Can you work these out from the model? Positions are in its coordinate system, mm. A direction names the side the tool comes from. Round coordinates to 2 decimals unless told otherwise and drop trailing zeros. Loops run counter-clockwise (first coordinate to the right, second up) from the corner with the lowest first, then second, coordinate; pieces in that order, holes last. Notation, with made-up numbers: (58, 23) -> (84, 23) arc R21 cw to (84, 60) -> close; hole circle Ø10 at (-2, 6). An arc over 180 degrees is marked (long way). Use a Markdown table: item, result.
from build123d import *

# Parameters (mm, degrees)
SKETCH_1_W          = 8
SKETCH_1_H          = 8
EXTRUDE_1_DEPTH     = 8
CUT_EXTRUDE_1_DEPTH = 8
SKETCH_3_R          = 3
EXTRUDE_2_DEPTH     = 60


with BuildPart() as part:
    # 草图1 → 凸台-拉伸1 (new body)
    with BuildSketch(Plane(origin=(0, 0, 0), x_dir=(1, 0, 0), z_dir=(0, 1, 0))):
        Rectangle(SKETCH_1_W, SKETCH_1_H)
    extrude(amount=EXTRUDE_1_DEPTH)

    # 草图2 → 切除-拉伸1 (cut)
    with BuildSketch(Plane.XY.offset(4)):
        with BuildLine():
            Line((-4, 4), (-4, 9.423328326))
            Line((-4, 9.423328326), (4, 9.423328326))
            Line((4, 9.423328326), (4, 4))
            ThreePointArc((4, 4), (0, 8), (-4, 4))
        make_face()
    extrude(amount=-CUT_EXTRUDE_1_DEPTH, mode=Mode.SUBTRACT)

    # 草图3 → 凸台-拉伸2 (add)
    with BuildSketch(Plane.XZ):
        Circle(SKETCH_3_R)
    extrude(amount=EXTRUDE_2_DEPTH)


solid = part.part
1. I need wall thicknesses on line 1 (Y direction, x = 0, z = 3.75); line 2 (Y direction, x = -0.25, z = -2.5); line 3 (Z direction, x = 1, y = -22.5). Which ranges of each line are inside material? Lowest first, please.
Answer sheet:
| item | result |
|---|---|
| line 1 | y = 0 to 8 |
| line 2 | y = -60 to 7.99 |
| line 3 | z = -2.83 to 2.83 |
2. Which directions (+Z, -Z, +X, -X, +Y, -Y) give clear straight access to the entire face, cutting with the end or side of a thin tool? Please do faces 1 (the flat face through (0, 4, -4)), 2 (the flat face through (2, 0, -3)).
Answer sheet:
| item | result |
|---|---|
| face 1 | -Z, +X, -X, +Y, -Y |
| face 2 | -Y |
3. I want a section at B-B (y = -48). Please give me the cut outline in (x, z).
Answer sheet:
| item | result |
|---|---|
| outline | circle Ø6 at (0, 0) |
4. I want a section at C-C (x = 0.75). Please give me the cut outline in (y, z).
Answer sheet:
| item | result |
|---|---|
| outline | (-60, -2.9) -> (0, -2.9) -> (0, -4) -> (7.93, -4) -> (7.93, 4) -> (0, 4) -> (0, 2.9) -> (-60, 2.9) -> close |
5. Will these pins go through, and if not, where does the flat tip stop? pin 1 Ø3 at (x, y) = (2, -35.5) entering from -Z; pin 2 Ø1 at (x, y) = (3, -49.5) entering from -Z.
Answer sheet:
| item | result |
|---|---|
| pin 1 | stops at z = -2.96 |
| pin 2 | stops at z = -1.66 |
6. I want a section at A-A (z = 0). Please give me the cut outline in (x, y), plus the area to 3 significant figures.
Answer sheet:
| item | result |
|---|---|
| outline | (-4, 0) -> (-3, 0) -> (-3, -60) -> (3, -60) -> (3, 0) -> (4, 0) -> (4, 4) arc R4 ccw to (-4, 4) -> close |
| area | 417 mm² |
